from build123d import *

# Parameters (mm, degrees)
F1_DEPTH    = 1.27
F3_D        = 2.54
F3_DEPTH    = 6.35
F3_TIP      = 0.7630929862
F4_R        = 1.524
F6_D        = 1.27
F6_DEPTH    = 6.35
F6_TIP      = 0.3815464931
F7_T1_DEPTH = 1.27
F9_D        = 13.843
F9_DEPTH    = 304.8
F9_TIP      = 4.1588567746


# Not quite as in the source:
# - a fillet or chamfer that OpenCascade refuses, or shapes differently, is made with other operations: its cross-section is extruded or revolved along the edge and cut away or added


with BuildPart() as f1:
    # F0 (on Front) → F1 (new body)
    with BuildSketch(Plane.XZ):
        with BuildLine():
            ThreePointArc((1.4341250062, 5.3522273875), (2.4839773751, 4.3023750186), (2.8682500124, 2.8682500124))
            Line((2.8682500124, 2.8682500124), (2.8682500124, 25.4276227206))
            Line((2.8682500124, 25.4276227206), (0, 25.4276227206))
            Line((0, 25.4276227206), (-1.4341250062, 25.4276227206))
            Line((-1.4341250062, 25.4276227206), (-2.8682500124, 25.4276227206))
            Line((-2.8682500124, 25.4276227206), (-2.8682500124, 2.8682500124))
            ThreePointArc((-2.8682500124, 2.8682500124), (-2.4839773751, 4.3023750186), (-1.4341250062, 5.3522273875))
            Line((-1.4341250062, 5.3522273875), (-1.4341250062, 22.6080268621))
            Line((-1.4341250062, 22.6080268621), (1.4341250062, 22.6080268621))
            Line((1.4341250062, 22.6080268621), (1.4341250062, 5.3522273875))
        make_face()
        with BuildLine():
            ThreePointArc((-2.8682500124, 2.8682500124), (0, 0), (2.8682500124, 2.8682500124))
            ThreePointArc((2.8682500124, 2.8682500124), (2.4839773751, 4.3023750186), (1.4341250062, 5.3522273875))
            ThreePointArc((1.4341250062, 5.3522273875), (0, 5.7365000248), (-1.4341250062, 5.3522273875))
            ThreePointArc((-1.4341250062, 5.3522273875), (-2.4839773751, 4.3023750186), (-2.8682500124, 2.8682500124))
        make_face()
    extrude(amount=F1_DEPTH)

    # F3
    with Locations(Plane(origin=(0, 0, 0), x_dir=(-1, 0, 0), z_dir=(0, 1, 0))):
        with Locations((0, 2.8682500124)):
            Hole(F3_D / 2, depth=F3_DEPTH)
            with Locations((0, 0, -(F3_DEPTH + F3_TIP / 2))):  # 118° drill point
                Cone(0, F3_D / 2, F3_TIP, mode=Mode.SUBTRACT)

    # F4
    f4_edges = [f1.edges().sort_by_distance(p)[0] for p in [
        (2.86825, -0.635, 25.427623),
        (-2.86825, -0.635, 25.427623),
    ]]
    fillet(f4_edges, radius=F4_R)

    # F6
    with Locations(Plane.XZ.offset(1.27)):
        with Locations((-1.5970880988, 24.1730304042), (0, 23.7946401586), (1.5335635452, 24.1730304042)):
            Hole(F6_D / 2, depth=F6_DEPTH)
            with Locations((0, 0, -(F6_DEPTH + F6_TIP / 2))):  # 118° drill point
                Cone(0, F6_D / 2, F6_TIP, mode=Mode.SUBTRACT)

    # F7: fillet of radius 1.905 on 2 edges, made by hand

    # F7_s2 → F7_t1 (join)
    with BuildSketch(Plane.XZ):
        with BuildLine():
            ThreePointArc((-0.4708749938, 22.6080268621), (0.8761634244, 22.0500652803), (1.4341250062, 20.7030268621))
            Line((1.4341250062, 20.7030268621), (1.4341250062, 22.6080268621))
            Line((1.4341250062, 22.6080268621), (-0.4708749938, 22.6080268621))
        make_face()
        with BuildLine():
            ThreePointArc((-1.4341250062, 20.7030268621), (-0.8761634244, 22.0500652803), (0.4708749938, 22.6080268621))
            Line((0.4708749938, 22.6080268621), (-1.4341250062, 22.6080268621))
            Line((-1.4341250062, 22.6080268621), (-1.4341250062, 20.7030268621))
        make_face()
    extrude(amount=F7_T1_DEPTH)

    # F9
    with Locations(Plane.XY.offset(25.4276227206)):
        with Locations((0, 6.6013582982)):
            Hole(F9_D / 2, depth=F9_DEPTH)
            with Locations((0, 0, -(F9_DEPTH + F9_TIP / 2))):  # 118° drill point
                Cone(0, F9_D / 2, F9_TIP, mode=Mode.SUBTRACT)


solid = f1.part
Could you check a few things on this model? Use its own coordinates, in mm. A direction names the side the tool comes from. Give positions to 0.01 mm unless a question says otherwise; leave off trailing zeros. Order: outer loops, then holes, each group sorted by start corner. A loop starts at its lowest first (then second) coordinate and runs counter-clockwise, first axis right, second up.
1. Will this pin go through, and if not, where does the flat tip stop? P1, Ø2, axis at x = -1.6, z = 24.17, coming from the +Y side.
2. Suppose I cut it at C-C (z = 4.5). List the corners of the cut face in (x, y) for me.
3. We'd pull the mould along X, two halves only. Please class faces 3 (the flat face through (2, -1.27, 10)), 4 (the cylindrical face through (-1.27, -0.74, 2.92)), 5 (the cylindrical face through (0, -1, 0)), 6 (the cylindrical face through (1.02, -0.71, 21.89)): pulls with the +X half, pulls with the -X half, needs draft (parallel to the pull), parting line crosses it, or undercut.
4. For faces 1 (the cylindrical face through (-1.044, -0.712, 21.858)), 2 (the cylindrical face through (-2.4, -0.6, 25)), which set-ups out of +Z, -Z, +X, -X, +Y, -Y let a thin tool reach every point of the face, with its end or its side?
5. Suppose I cut it at B-B (y = -0.6). List the corners of the cut face in (x, z) for me (1 decimal), plus the area to 3 significant figures.
6. I need wall thicknesses on L1, parallel to X at y = -1.05, z = 19.25; L2, parallel to Z at x = -0.8, y = -0.6; L3, parallel to Z at x = 0.75, y = -0.55. Which ranges of each line are inside material? Lowest first, please.
7. Suppose I cut it at A-A (z = 16.5). List the corners of the cut face in (x, y) for me.
Solved:
1. P1: stops at y = 0
2. outline: (-2.87, -1.27) - (2.87, -1.27) - (2.87, 0) - (2.08, 0) arc R6.92 cw to (-2.08, 0) - (-2.87, 0) - close
3. face 3: needs draft
3. face 4: undercut
3. face 5: parting line crosses it
3. face 6: undercut
4. face 1: +Y, -Y
4. face 2: +Z, -X, +Y, -Y
5. outline: (-2.9, 2.9) arc R2.9 ccw to (2.9, 2.9) - (2.9, 23.9) arc R1.5 ccw to (1.3, 25.4) - (-1.3, 25.4) arc R1.5 ccw to (-2.9, 23.9) - close; hole circle Ø1.3 at (-1.6, 24.2); hole (-1.4, 5.4) arc R2.9 cw to (1.4, 5.4) - (1.4, 20.7) arc R1.9 ccw to (0, 22.5) arc R1.9 ccw to (-1.4, 20.7) - close; hole circle Ø2.5 at (0, 2.9); hole circle Ø1.3 at (0, 23.8); hole circle Ø1.3 at (1.5, 24.2)
5. area: 85.3 mm2
6. L1: x = -2.87 to -1.43, 1.43 to 2.87
6. L2: z = 0.11 to 1.88, 3.85 to 5.62, 22.12 to 25.43
6. L3: z = 0.1 to 1.84, 3.89 to 5.64, 22.17 to 25.43
7. outline: (-2.87, -1.27) - (-1.43, -1.27) - (-1.43, -0.17) arc R6.92 cw to (-2.08, 0) - (-2.87, 0) - close; (1.43, -1.27) - (2.87, -1.27) - (2.87, 0) - (2.08, 0) arc R6.92 cw to (1.43, -0.17) - close
